Input: part model. Units: mm. Frame: model coordinates. Face numbers are marked on the shaded views. Give positions to 0.01 mm unless a question says otherwise; leave off trailing zeros. Loops run counter-clockwise (first coordinate to the right, second up) from the corner with the lowest first, then second, coordinate; pieces in that order, holes last. Notation, with made-up numbers: M -34,68.5 L 11,68.5 A21 ccw 11,79.5 Z; hole C 50,-30 d11. An arc over 180 degrees is marked long. Answer as a JSON object with one key per item and string values. Group by question number.
1) Section query B-B on z = -39. Return loops of the section in (x, y), plus the area to 3 significant figures.
2) Ray query, L1, parallel to Z at x = -35, y = -57.5; L2, parallel to X at y = -159, z = 48; L3, parallel to Z at x = -48, y = -225. Return the intervals inside material, ascending.
3) First-contact query: P1, Ø14, axis at y = 25, z = 110, coming from the +X side; P2, Ø19.5, axis at x = -14, y = -151, coming from the +Z side; P3, Ø15.5, axis at y = 125, z = -110, coming from the -X side; P4, Ø1.5, axis at y = -135, z = -78, coming from the -X side. Flat tips, straight axial feed; report the tip coordinate or a pass-through.
4) Draft query along Z for the marked faces 1, 2, 3 and 4. Return one class per face: +Z half, -Z half, draft (parallel to the pull), parting line (faces both ways), or undercut.
5) Section query D-D on z = 110. Count the separate pieces of the cut face and the enclosed holes in it, plus the area to 3 significant figures.
6) Section query C-C on y = 103. Return loops of the section in (x, z).
7) Section query A-A on x = -18.5. Return loops of the section in (y, z), plus the area to 3 significant figures.
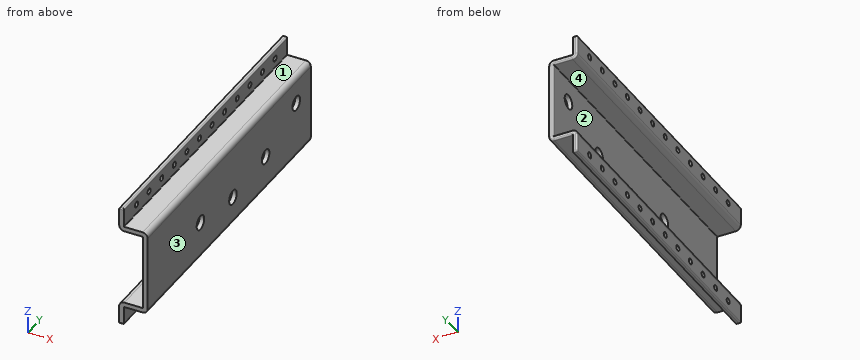
from build123d import *

# Parameters (mm, degrees)
SKETCH1_W                       = 180
SKETCH1_H                       = 650
BASE_FLANGE1_DEPTH              = 10
EDGE_FLANGE1_STRIP_W            = 41.4732
EDGE_FLANGE1_STRIP_H            = 10
EDGE_FLANGE1_STRIP_CUT_DEPTH    = 650
EDGE_FLANGE1_STRIP_2_W          = 41.4732
EDGE_FLANGE1_STRIP_2_H          = 10
EDGE_FLANGE1_STRIP_CUT_2_DEPTH  = 650
EDGE_FLANGE1_DEPTH              = 650
EDGE_FLANGE1_BEND_DEPTH         = 650
EDGE_FLANGE2_STRIP_W            = 41.4732
EDGE_FLANGE2_STRIP_H            = 10
EDGE_FLANGE2_STRIP_CUT_DEPTH    = 650
EDGE_FLANGE2_STRIP_2_W          = 41.4732
EDGE_FLANGE2_STRIP_2_H          = 10
EDGE_FLANGE2_STRIP_CUT_2_DEPTH  = 650
EDGE_FLANGE2_DEPTH              = 650
EDGE_FLANGE2_BEND_DEPTH         = 650
SKETCH18_R                      = 15
CUT_EXTRUDE1_DEPTH              = 10
M10_CLEARANCE_HOLE1_D           = 12
M10_CLEARANCE_HOLE1_CSINK_D     = 12.05
M10_CLEARANCE_HOLE1_CSINK_ANGLE = 90
FILLET1_R                       = 3


# Sheet-metal steps are written as plain solids
with BuildPart() as part:
    # Sketch1 → Base-Flange1 (new body)
    with BuildSketch(Plane(origin=(0, 0, 0), x_dir=(0, 0, -1), z_dir=(1, 0, 0))):
        Rectangle(SKETCH1_W, SKETCH1_H)
    extrude(amount=BASE_FLANGE1_DEPTH)

    # Edge-Flange1 strip (across the edge) → Edge-Flange1 strip cut (cut)
    with BuildSketch(Plane(origin=(0, -325, 90), x_dir=(0, 0, -1), z_dir=(0, 1, 0))):
        with Locations((-10, -5)):
            Rectangle(EDGE_FLANGE1_STRIP_W, EDGE_FLANGE1_STRIP_H)
    extrude(amount=EDGE_FLANGE1_STRIP_CUT_DEPTH, mode=Mode.SUBTRACT)

    # Edge-Flange1 strip 2 (across the edge) → Edge-Flange1 strip cut 2 (cut)
    with BuildSketch(Plane(origin=(0, 325, -90), x_dir=(0, 0, 1), z_dir=(0, -1, 0))):
        with Locations((-10, -5)):
            Rectangle(EDGE_FLANGE1_STRIP_2_W, EDGE_FLANGE1_STRIP_2_H)
    extrude(amount=EDGE_FLANGE1_STRIP_CUT_2_DEPTH, mode=Mode.SUBTRACT)

    # Edge-Flange1 section (across the edge) → Edge-Flange1 (add)
    with BuildSketch(Plane(origin=(0, -325, 90), x_dir=(0, 0, -1), z_dir=(0, 1, 0))):
        with BuildLine():
            Line((0, 0.7366), (0, 50))
            Line((0, 50), (10, 50))
            Line((10, 50), (10, 0.7366))
            ThreePointArc((10, 0.7366), (10.215745145, 0.215745145), (10.7366, 0))
            Line((10.7366, 0), (10.7366, -10))
            ThreePointArc((10.7366, -10), (3.144677333, -6.855322667), (0, 0.7366))
        make_face()
    extrude(amount=EDGE_FLANGE1_DEPTH)

    # Edge-Flange1 section 2 (across the edge) → Edge-Flange1 bend (add)
    with BuildSketch(Plane(origin=(0, 325, -90), x_dir=(0, 0, 1), z_dir=(0, -1, 0))):
        with BuildLine():
            Line((0, 0.7366), (0, 50))
            Line((0, 50), (10, 50))
            Line((10, 50), (10, 0.7366))
            ThreePointArc((10, 0.7366), (10.215745145, 0.215745145), (10.7366, 0))
            Line((10.7366, 0), (10.7366, -10))
            ThreePointArc((10.7366, -10), (3.144677333, -6.855322667), (0, 0.7366))
        make_face()
    extrude(amount=EDGE_FLANGE1_BEND_DEPTH)

    # Edge-Flange2 strip (across the edge) → Edge-Flange2 strip cut (cut)
    with BuildSketch(Plane(origin=(-50, 325, 90), x_dir=(1, 0, 0), z_dir=(0, -1, 0))):
        with Locations((-10, -5)):
            Rectangle(EDGE_FLANGE2_STRIP_W, EDGE_FLANGE2_STRIP_H)
    extrude(amount=EDGE_FLANGE2_STRIP_CUT_DEPTH, mode=Mode.SUBTRACT)

    # Edge-Flange2 strip 2 (across the edge) → Edge-Flange2 strip cut 2 (cut)
    with BuildSketch(Plane(origin=(-50, -325, -90), x_dir=(1, 0, 0), z_dir=(0, 1, 0))):
        with Locations((-10, -5)):
            Rectangle(EDGE_FLANGE2_STRIP_2_W, EDGE_FLANGE2_STRIP_2_H)
    extrude(amount=EDGE_FLANGE2_STRIP_CUT_2_DEPTH, mode=Mode.SUBTRACT)

    # Edge-Flange2 section (across the edge) → Edge-Flange2 (add)
    with BuildSketch(Plane(origin=(-50, 325, 90), x_dir=(1, 0, 0), z_dir=(0, -1, 0))):
        with BuildLine():
            Line((0, 0.7366), (0, 40))
            Line((0, 40), (10, 40))
            Line((10, 40), (10, 0.7366))
            ThreePointArc((10, 0.7366), (10.215745145, 0.215745145), (10.7366, 0))
            Line((10.7366, 0), (10.7366, -10))
            ThreePointArc((10.7366, -10), (3.144677333, -6.855322667), (0, 0.7366))
        make_face()
    extrude(amount=EDGE_FLANGE2_DEPTH)

    # Edge-Flange2 section 2 (across the edge) → Edge-Flange2 bend (add)
    with BuildSketch(Plane(origin=(-50, -325, -90), x_dir=(1, 0, 0), z_dir=(0, 1, 0))):
        with BuildLine():
            Line((0, 0.7366), (0, 40))
            Line((0, 40), (10, 40))
            Line((10, 40), (10, 0.7366))
            ThreePointArc((10, 0.7366), (10.215745145, 0.215745145), (10.7366, 0))
            Line((10.7366, 0), (10.7366, -10))
            ThreePointArc((10.7366, -10), (3.144677333, -6.855322667), (0, 0.7366))
        make_face()
    extrude(amount=EDGE_FLANGE2_BEND_DEPTH)

    # Sketch18 → Cut-Extrude1 (cut)
    with BuildSketch(Plane(origin=(10, 0, 0), x_dir=(0, 0, -1), z_dir=(1, 0, 0))):
        with Locations(Location((-31.365756011, 265, 0), (0, 0, 180))):
            Circle(SKETCH18_R)
        with Locations(Location((15.804715389, 143.295302131, 0), (0, 0, 180))):
            Circle(SKETCH18_R)
        with Locations(Location((29.868398264, 13.528974914, 0), (0, 0, 180))):
            Circle(SKETCH18_R)
        with Locations(Location((9.86687587, -115.455620901, 0), (0, 0, 180))):
            Circle(SKETCH18_R)
    extrude(amount=-CUT_EXTRUDE1_DEPTH, mode=Mode.SUBTRACT)

    # M10 Clearance Hole1 (through all)
    with Locations(Plane(origin=(-40, 0, 0), x_dir=(0, 0, -1), z_dir=(1, 0, 0))):
        with Locations((-110, -275), (-110, -225), (-110, -175), (-110, -125), (-110, -75), (-110, -25), (-110, 25), (-110, 75), (-110, 125), (-110, 175), (-110, 225), (-110, 275)):
            m10_clearance_hole1 = CounterSinkHole(M10_CLEARANCE_HOLE1_D / 2, M10_CLEARANCE_HOLE1_CSINK_D / 2, counter_sink_angle=M10_CLEARANCE_HOLE1_CSINK_ANGLE)

    # Mirror1: M10 Clearance Hole1 across plane
    add(m10_clearance_hole1.mirror(Plane.XY), mode=Mode.SUBTRACT)

    # Fillet1
    fillet1_edges = [part.edges().sort_by_distance(p)[0] for p in [
        (-46.855322667, 325, 83.144677333),
        (-39.784254855, 325, 90.215745145),
        (-45, 325, 130),
        (-40, 325, 110.3683),
        (-50, 0, 130),
        (-50, 325, 110.3683),
        (-40, 0, 130),
        (-45, -325, 130),
        (-46.855322667, 325, -83.144677333),
        (-39.784254855, 325, -90.215745145),
        (-45, -325, -130),
        (-40, 325, -110.3683),
        (-50, 325, -110.3683),
        (-50, 0, -130),
        (-40, 0, -130),
        (-45, 325, -130),
        (0, 325, 0),
        (10, 325, 0),
        (6.855322667, 325, 86.855322667),
        (-0.215745145, 325, 79.784254855),
        (-20, 325, 80),
        (-20, 325, 90),
        (6.855322667, 325, -86.855322667),
        (-0.215745145, 325, -79.784254855),
        (-20, 325, -80),
        (-20, 325, -90),
    ]]
    fillet(fillet1_edges, radius=FILLET1_R)


solid = part.part
Output:
{
 "1": {"outline": "M 0,-325 L 10,-325 L 10,1.63 L 0,1.63 Z; M 0,25.43 L 10,25.43 L 10,322 A3 ccw 7,325 L 3,325 A3 ccw 0,322 Z", "area": "6,260 mm^2"},
 "2": {"L1": "z = -90 to -80, 80 to 90", "L2": "x = 0 to 10", "L3": "z = -129.83 to -116, -104 to -84.5, 84.5 to 104, 116 to 129.83"},
 "3": {"P1": "stops at x = -40", "P2": "stops at z = 90", "P3": "stops at x = -50", "P4": "stops at x = 0"},
 "4": {"face 1": "+Z half", "face 2": "undercut", "face 3": "draft", "face 4": "undercut"},
 "5": {"separate pieces": "13", "enclosed holes": "0", "area": "5,060 mm^2"},
 "6": {"outline": "M -50,-127 A3 ccw -47,-130 L -43,-130 A3 ccw -40,-127 L -40,-90.74 A0.74 cw -39.26,-90 L -0.74,-90 A10.74 ccw 10,-79.26 L 10,79.26 A10.74 ccw -0.74,90 L -39.26,90 A0.74 cw -40,90.74 L -40,127 A3 ccw -43,130 L -47,130 A3 ccw -50,127 L -50,90.74 A10.74 ccw -39.26,80 L -0.74,80 A0.74 cw 0,79.26 L 0,-79.26 A0.74 cw -0.74,-80 L -39.26,-80 A10.74 ccw -50,-90.74 Z"},
 "7": {"outline": "M -325,-90 L 322,-90 A3 ccw 325,-87 L 325,-83 A3 ccw 322,-80 L -325,-80 Z; M -325,80 L 322,80 A3 ccw 325,83 L 325,87 A3 ccw 322,90 L -325,90 Z", "area": "13,000 mm^2"}
}
